from build123d import *

# Parameters (mm, degrees)
SKETCH1_W                = 75.15
SKETCH1_H                = 75.15
SKETCH1_W_2              = 14
SKETCH1_H_2              = 14
BOSS_EXTRUDE1_DEPTH      = 3
SKETCH2_R                = 1
CUT_EXTRUDE1_DEPTH       = 3
CHAMFER1_SIZE            = 1
CHAMFER1_OF_MIRROR1_SIZE = 1
MOVE_FACE1_BY            = 0.2
MOVE_FACE1_2_BY          = 0.2
MOVE_FACE1_3_BY          = 0.2
MOVE_FACE1_4_BY          = 0.2
FILLET1_R                = 2


with BuildPart() as part:
    # Sketch1 → Boss-Extrude1 (new body)
    with BuildSketch(Plane(origin=(0, 0, 0), x_dir=(1, 0, 0), z_dir=(0, 1, 0))):
        Rectangle(SKETCH1_W, SKETCH1_H)
        with Locations((-9.525, 28.575)):
            Rectangle(SKETCH1_W_2, SKETCH1_H_2, mode=Mode.SUBTRACT)
        with Locations((-28.575, 28.575)):
            Rectangle(SKETCH1_W_2, SKETCH1_H_2, mode=Mode.SUBTRACT)
        with Locations((9.525, 28.575)):
            Rectangle(SKETCH1_W_2, SKETCH1_H_2, mode=Mode.SUBTRACT)
        with Locations((28.575, 28.575)):
            Rectangle(SKETCH1_W_2, SKETCH1_H_2, mode=Mode.SUBTRACT)
        with Locations((-9.525, 9.525)):
            Rectangle(SKETCH1_W_2, SKETCH1_H_2, mode=Mode.SUBTRACT)
        with Locations((9.525, 9.525)):
            Rectangle(SKETCH1_W_2, SKETCH1_H_2, mode=Mode.SUBTRACT)
        with Locations((28.575, 9.525)):
            Rectangle(SKETCH1_W_2, SKETCH1_H_2, mode=Mode.SUBTRACT)
        with Locations((-9.525, -9.525)):
            Rectangle(SKETCH1_W_2, SKETCH1_H_2, mode=Mode.SUBTRACT)
        with Locations((9.525, -9.525)):
            Rectangle(SKETCH1_W_2, SKETCH1_H_2, mode=Mode.SUBTRACT)
        with Locations((28.575, -9.525)):
            Rectangle(SKETCH1_W_2, SKETCH1_H_2, mode=Mode.SUBTRACT)
        with Locations((-9.525, -28.575)):
            Rectangle(SKETCH1_W_2, SKETCH1_H_2, mode=Mode.SUBTRACT)
        with Locations((9.525, -28.575)):
            Rectangle(SKETCH1_W_2, SKETCH1_H_2, mode=Mode.SUBTRACT)
        with Locations((28.575, -28.575)):
            Rectangle(SKETCH1_W_2, SKETCH1_H_2, mode=Mode.SUBTRACT)
        with Locations((-28.575, 9.525)):
            Rectangle(SKETCH1_W_2, SKETCH1_H_2, mode=Mode.SUBTRACT)
        with Locations((-28.575, -9.525)):
            Rectangle(SKETCH1_W_2, SKETCH1_H_2, mode=Mode.SUBTRACT)
        with Locations((-28.575, -28.575)):
            Rectangle(SKETCH1_W_2, SKETCH1_H_2, mode=Mode.SUBTRACT)
    extrude(amount=BOSS_EXTRUDE1_DEPTH)

    # Sketch2 → Cut-Extrude1 (cut)
    with BuildSketch(Plane(origin=(0, 3, 0), x_dir=(1, 0, 0), z_dir=(0, 1, 0))):
        with Locations(Location((-19.05, 19.05, 0), (0, 0, 270))):
            Circle(SKETCH2_R)
        with Locations(Location((-28.575, -19.05, 0), (0, 0, 270))):
            Circle(SKETCH2_R)
    cut_extrude1 = extrude(amount=-CUT_EXTRUDE1_DEPTH, mode=Mode.SUBTRACT)

    # Chamfer1
    chamfer1_edges = [part.edges().sort_by_distance(p)[0] for p in [
        (-19.05, 3, -20.05),
        (-28.575, 3, 18.05),
    ]]
    chamfer(chamfer1_edges, length=CHAMFER1_SIZE)

    # Mirror1: Cut-Extrude1 across plane
    add(cut_extrude1.mirror(Plane(origin=(0, 0, 0), x_dir=(0, 0, 1), z_dir=(1, 0, 0))), mode=Mode.SUBTRACT)

    # Chamfer1 of Mirror1
    chamfer1_of_mirror1_edges = [part.edges().sort_by_distance(p)[0] for p in [
        (19.05, 3, -20.05),
        (28.575, 3, 18.05),
    ]]
    chamfer(chamfer1_of_mirror1_edges, length=CHAMFER1_OF_MIRROR1_SIZE)

    # Move Face1: a face moved inward by 0.2
    extrude(part.faces().sort_by_distance((37.575, 1.5, 0))[0], amount=MOVE_FACE1_BY, dir=(-1, 0, 0), mode=Mode.SUBTRACT)

    # Move Face1 2: a face moved inward by 0.2
    extrude(part.faces().sort_by_distance((0, 1.5, -37.575))[0], amount=MOVE_FACE1_2_BY, dir=(0, 0, 1), mode=Mode.SUBTRACT)

    # Move Face1 3: a face moved inward by 0.2
    extrude(part.faces().sort_by_distance((0, 1.5, 37.575))[0], amount=MOVE_FACE1_3_BY, dir=(0, 0, -1), mode=Mode.SUBTRACT)

    # Move Face1 4: a face moved inward by 0.2
    extrude(part.faces().sort_by_distance((-37.575, 1.5, 0))[0], amount=MOVE_FACE1_4_BY, dir=(1, 0, 0), mode=Mode.SUBTRACT)

    # Fillet1
    fillet1_edges = [part.edges().sort_by_distance(p)[0] for p in [
        (37.375, 1.5, 37.375),
        (-37.375, 1.5, 37.375),
        (-37.375, 1.5, -37.375),
        (37.375, 1.5, -37.375),
    ]]
    fillet(fillet1_edges, radius=FILLET1_R)


solid = part.part
The model under review builds one solid part; all positions refer to its coordinate system, in mm. A direction names the side the tool comes from. Round coordinates to 2 decimals unless told otherwise and drop trailing zeros. Loops run counter-clockwise (first coordinate to the right, second up) from the corner with the lowest first, then second, coordinate; pieces in that order, holes last. Notation, with made-up numbers: (35, 66) - (59, 66) arc R14 ccw to (59, 79) - close; hole circle Ø2 at (80.5, 23). An arc over 180 degrees is marked (long way). Use CSV: the item, a comma, the result in double quotes.
(1) Take a section at A-A, the plane z = 29.5. Give the boundary of the cut face in (x, y) (3 decimals).
Working result:
outline,"(-37.375, 0) - (-35.575, 0) - (-35.575, 3) - (-37.375, 3) - close; (-21.575, 0) - (-16.525, 0) - (-16.525, 3) - (-21.575, 3) - close; (-2.525, 0) - (2.525, 0) - (2.525, 3) - (-2.525, 3) - close; (16.525, 0) - (21.575, 0) - (21.575, 3) - (16.525, 3) - close; (35.575, 0) - (37.375, 0) - (37.375, 3) - (35.575, 3) - close"
(2) Take a section at D-D, the plane z = 19.05. Give the boundary of the cut face in (x, y) (3 decimals).
Working result:
outline,"(-37.375, 0) - (-29.575, 0) - (-29.575, 2) - (-30.575, 3) - (-37.375, 3) - close; (-27.575, 0) - (27.575, 0) - (27.575, 2) - (26.575, 3) - (-26.575, 3) - (-27.575, 2) - close; (29.575, 0) - (37.375, 0) - (37.375, 3) - (30.575, 3) - (29.575, 2) - close"
(3) Take a section at C-C, the plane x = -25. Give the boundary of the cut face in (y, z) (3 decimals), plus the area to 4 significant figures.
Working result:
outline,"(0, -37.375) - (3, -37.375) - (3, -35.575) - (0, -35.575) - close; (0, -21.575) - (3, -21.575) - (3, -16.525) - (0, -16.525) - close; (0, -2.525) - (3, -2.525) - (3, 2.525) - (0, 2.525) - close; (0, 16.525) - (3, 16.525) - (3, 21.575) - (0, 21.575) - close; (0, 35.575) - (3, 35.575) - (3, 37.375) - (0, 37.375) - close"
area,"56.25 mm^2"
(4) For line 1 (Z direction, x = -24, y = 0.55) (3 decimals); line 2 (X direction, y = 1.85, z = 19) (3 decimals); line 3 (X direction, y = 0.8, z = -19.05) (3 decimals), list the stretches that pass through material, from the lowest coordinate up.
Working result:
line 1,"z = -37.375 to -35.575, -21.575 to -16.525, -2.525 to 2.525, 16.525 to 21.575, 35.575 to 37.375"
line 2,"x = -37.375 to -29.574, -27.576 to 27.576, 29.574 to 37.375"
line 3,"x = -37.375 to -20.05, -18.05 to 18.05, 20.05 to 37.375"
(5) Clearance check with flat-ended pins moving along their axes: P1, Ø2, axis at x = -7.5, z = 23, coming from the -Y side; P2, Ø2.5, axis at x = -28.575, z = 19.05, coming from the +Y side. State where each tip first meets the part, or that it passes through.
Working result:
P1,"passes through"
P2,"stops at y = 2.25"
(6) The part is to be moulded in two halves that separate along Z. For faces 3 (the flat face through (21.575, 1, 29)), 4 (the flat face through (37.375, 1, 0)), say which applies: pulls with the +Z half, pulls with the -Z half, needs draft (parallel to the pull), parting line crosses it, or undercut.
Working result:
face 3,"undercut"
face 4,"needs draft"
(7) Machinability: for faces 1 (the flat face through (-1, 3, -1)), 2 (the flat face through (2.525, 1, -9)), which of the approach directions +Z, -Z, +X, -X, +Y, -Y give a long, thin tool a straight path to every point of the face, cutting with its end or side? Answer none if there is none.
Working result:
face 1,"+Z, -Z, +X, -X, +Y"
face 2,"+Y, -Y"
(8) Take a section at B-B, the plane x = 19.05. Give the boundary of the cut face in (y, z) (3 decimals), plus the area to 3 significant figures.
Working result:
outline,"(0, -37.375) - (3, -37.375) - (3, -21.05) - (2, -20.05) - (0, -20.05) - close; (0, -18.05) - (2, -18.05) - (3, -17.05) - (3, 37.375) - (0, 37.375) - close"
area,"217 mm^2"
